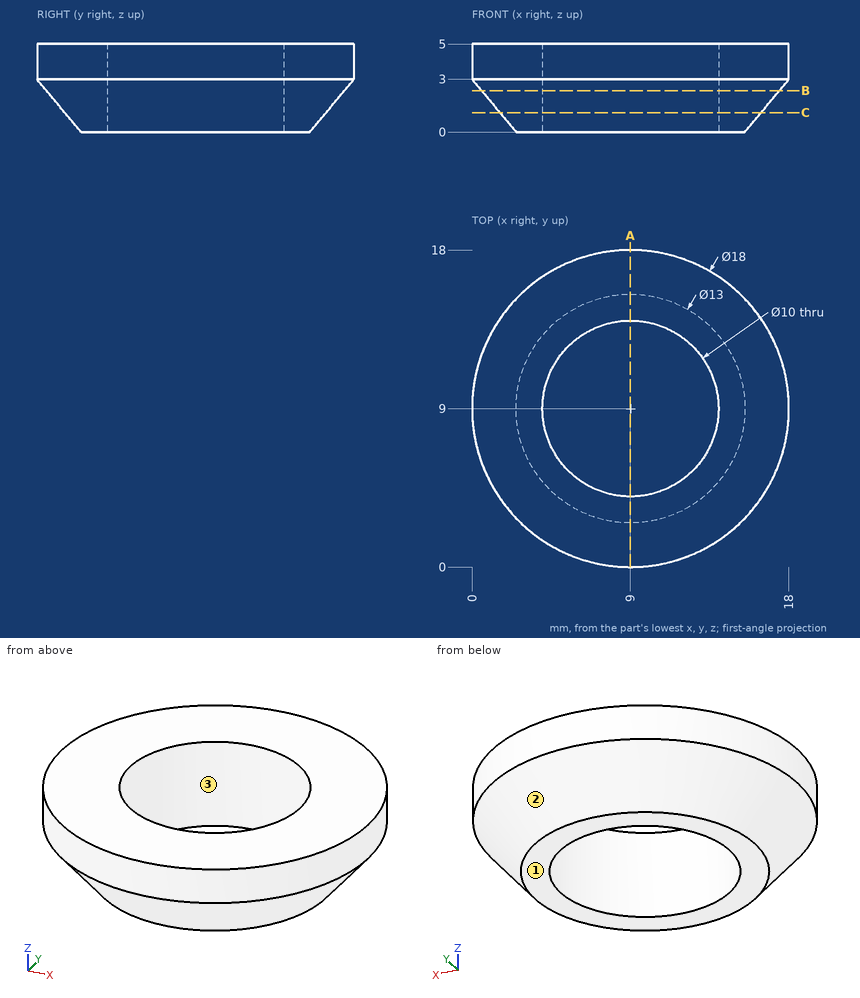
Job drawing, mm, ordinate dimensions from the low corner. One solid piece. Give positions to 0.01 mm unless a question says otherwise; leave off trailing zeros. Loops run counter-clockwise (first coordinate to the right, second up) from the corner with the lowest first, then second, coordinate; pieces in that order, holes last. Notation, with made-up numbers: (-14.5, 37) -> (37.5, 37) arc R19 cw to (37.5, 59) -> close; hole circle Ø3 at (89, -39.5). An arc over 180 degrees is marked (long way). Write each question's results on one line, items separated by ' | '.
(1) Probe line 1 along Y through (x, z) = (9, 3.65); line 2 along Y through (x, z) = (9, 2); line 3 along X through (y, z) = (8.5, 4.3). List the from-to ranges inside material, lowest first.
Geometry results:
line 1: y = 0 to 4, 14 to 18 | line 2: y = 0.83 to 4, 14 to 17.17 | line 3: x = 0.01 to 4.03, 13.97 to 17.99
(2) Cut at B-B on z = 2.35. List the corners of the cut face in (x, y), and give its area (3 significant figures).
Geometry results:
outline: circle Ø16.92 at (9, 9); hole circle Ø10 at (9, 9) | area: 146 mm²
(3) Cut at C-C on z = 1.1. List the corners of the cut face in (x, y), and give its area (3 significant figures).
Geometry results:
outline: circle Ø14.83 at (9, 9); hole circle Ø10 at (9, 9) | area: 94.3 mm²
(4) Flat gauge pin, fed straight in: pin 1 Ø1.5 at (x, z) = (14.5, 3.5) entering from -Y. Where does the tip first touch, or does it go through?
Geometry results:
pin 1: stops at y = 1.36
(5) Cut at A-A on x = 9. List the corners of the cut face in (y, z), and give its area (3 significant figures).
Geometry results:
outline: (0, 3) -> (2.5, 0) -> (4, 0) -> (4, 5) -> (0, 5) -> close; (14, 0) -> (15.5, 0) -> (18, 3) -> (18, 5) -> (14, 5) -> close | area: 32.5 mm²
(6) Pull direction X, two halves, no side cores. Call the marked faces 1, 2 and 3: released by +X, released by -X, zero draft, split by the parting line, or undercut.
Geometry results:
face 1: zero draft | face 2: split by the parting line | face 3: undercut
